Read the model definition and answer for the solid it produces. Units are mm, in the model's axes. Face numbers are marked on the shaded views. A direction names the side the tool comes from. Coordinates: 2 decimals unless noted, no trailing zeros. Loops run counter-clockwise (first coordinate to the right, second up) from the corner with the lowest first, then second, coordinate; pieces in that order, holes last. Notation, with made-up numbers: M 3,71 L 46,71 A26 cw 46,106 Z; hole C 1.25,68.5 d9. An arc over 180 degrees is marked long. One line per item, written item: value. Start each with the question number.
1. For the marked faces 1, 2 and 3, determine the directions among +Z, -Z, +X, -X, +Y, -Y from which every point of the face is accessible in a straight line to the end or side of a thin tool.
2. Flat-ended cylindrical pins translate along their axes: pin 1 (12 mm diameter, centred on x = -22.5, y = -18, fed in from +Z); pin 2 (19.5 mm diameter, centred on y = -15.5, z = -32.5, fed in from +X); pin 3 (5.5 mm diameter, centred on y = -21, z = -36.37, fed in from -X); pin 4 (20 mm diameter, centred on y = 21, z = -36.37, fed in from -X). Find the tip coordinate at first contact, or state that the pin passes through.
3. The part is cut by section C-C (x = -22.5). Write down the section's boundary in (y, z).
4. The part is cut by section A-A (x = 3). Write down the section's boundary in (y, z).
5. Consider probe 1 along Y at (x, z) = (9.5, 0); probe 2 along Z at (x, y) = (8, -14); probe 3 along X at (y, z) = (-10.5, -45.5). Determine where each line is inside the solid, lowest interval first.
6. The part is cut by section B-B (z = 0). State how many separate pieces and enclosed holes the cut face has, then the cut area to 3 significant figures.
7. Determine the mould class of the marked faces 4, 5 and 6 for opening direction Y: +Y half, -Y half, draft (parallel to the pull), parting line (faces both ways), or undercut.
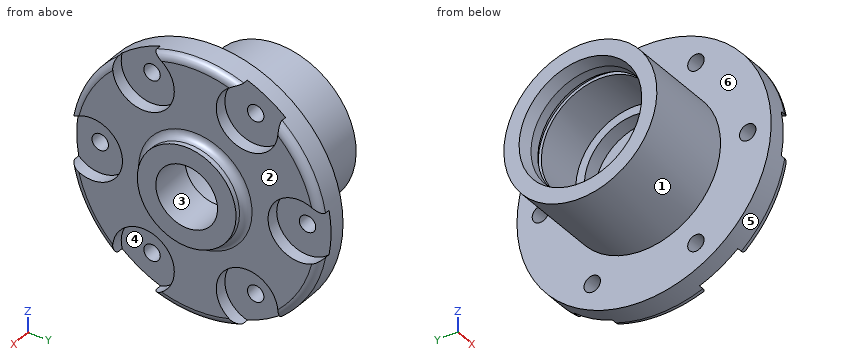
Autodesk Inventor part; units mm, degrees
ref_plane "Work Plane1" through (-26, 0, 0) normal (-1, 0, 0) x (0, 0, 1)
ref_plane "YZ Plane" through (0, 0, 0) normal (1, 0, 0) x (0, 1, 0)
ref_plane "XZ Plane" through (0, 0, 0) normal (0, 1, 0) x (-1, 0, 0)
sketch "Sketch1" plane through (0, 0, 0) normal (1, 0, 0) x (0, 1, 0)
  circle A0 centre (0, 0) radius 51.5
  circle A1 centre (0, 0) radius 31
  circle A2 centre (0, 0) radius 11
  dimension "d0" = 103
  dimension "d2" = 62
  dimension "d3" = 22
extrude "Extrusion1" add sketch "Sketch1" along normal blind 12 contours A0 | A1 | A2
sketch "Sketch3" plane through (0, 0, 0) normal (-1, 0, 0) x (0, 0, 1)
  circle A0 centre (0, 0) radius 11
  circle A1 centre (0, 0) radius 31
  dimension "d13" = 62
extrude "Extrusion2" add sketch "Sketch3" along normal blind 60 contours A0 | A1
sketch "Sketch4" plane through (12, 0, 0) normal (1, 0, 0) x (0, 0, -1)
  circle A0 centre (0, 0) radius 20
  dimension "d16" = 40
extrude "Extrusion3" add sketch "Sketch4" along normal blind 5
sketch "Sketch6" plane through (12, 0, 0) normal (1, 0, 0) x (0, 0, -1)
  circle A0 centre (0, 0) radius 11
  circle A1 centre (0, 0) radius 42
  line L0 (0, 0) -> (0, 42)
  point P0 (0.0095, 11)
  point P1 (0.0095, -11)
  point P2 (-36.3731, 21)
  point P3 (-36.3731, -21)
  point P4 (0, -42)
  point P5 (36.3731, -21)
  point P6 (36.3731, 21)
  dimension "d30" = 84
  dimension "d28" = 360
hole "Hole3" at (12, 42, 0) at (12, 21, 36.3731) at (12, -21, 36.3731) at (12, -42, 0) at (12, -21, -36.3731) at (12, 21, -36.3731) direction (-1, 0, 0) diameter 6.647 end through all counterbore diameter 25 counterbore depth 5
thread "Thread1"
sketch "Sketch7" plane through (17, 0, 0) normal (1, 0, 0) x (0, 0, -1)
  circle A0 centre (0, 0) radius 20
  circle A1 centre (0, 0) radius 12.5
  dimension "d40" = 25
extrude "Extrusion4" cut sketch "Sketch7" against normal blind 100 contours A1
fillet "Fillet1" radius 3 6 edges at (12, 44.6003, -25.75) (12, 0, -51.5) (12, -44.6003, -25.75) (12, -44.6003, 25.75) (12, 0, 51.5) (12, 44.6003, 25.75)
fillet "Fillet2" radius 3 1 edges at (12, 0, 20)
sketch "Sketch8" plane through (-60, 0, 0) normal (-1, 0, 0) x (0, 0, 1)
  circle A0 centre (0, 0) radius 23.5
  dimension "d45" = 47
extrude "Extrusion5" cut sketch "Sketch8" against normal blind 60
sketch "Sketch9" plane through (-60, 0, 0) normal (-1, 0, 0) x (0, 0, 1)
  circle A0 centre (0, 0) radius 11
  circle A1 centre (0, 0) radius 31
  circle A2 centre (0, 0) radius 31
extrude "Extrusion6" cut sketch "Sketch9" against normal blind 23 contours A0 | A1
chamfer "Chamfer1" distance 5 angle 15 1 edges at (-37, 0, -23.5) measured on face at (-12.3333, -1.891, 23.4238)
sketch "Sketch10" plane through (0, 0, 0) normal (-1, 0, 0) x (0, 0, 1)
  circle A0 centre (0, 0) radius 20
  circle A1 centre (0, 0) radius 23.5
  dimension "d60" = 40
extrude "Extrusion7" add sketch "Sketch10" along normal blind 6
ref_plane "Work Plane1" through (-26, 0, 0) normal (-1, 0, 0) x (0, 0, 1)
sketch "Sketch11" plane through (-26, 0, 0) normal (-1, 0, 0) x (0, 0, 1)
  circle A0 centre (0, 0) radius 24.75
  dimension "d64" = 49.5
extrude "Extrusion8" cut sketch "Sketch11" along normal blind 2
properties part number "END CAP" material "Iron, Cast"
Answer block:
1. face 1: -X
1. face 2: +X
1. face 3: +X, -X
2. pin 1: stops at z = 28.58
2. pin 2: stops at x = 12
2. pin 3: passes through
2. pin 4: stops at x = 0
3. outline: C 0,0 d62; hole C 0,0 d47
4. outline: C 0,0 d103; hole C -42,0 d6.65; hole C -21,-36.37 d6.65; hole C -21,36.37 d6.65; hole C 0,0 d25; hole C 21,-36.37 d6.65; hole C 21,36.37 d6.65; hole C 42,0 d6.65
5. probe 1: y = -29.5 to -12.5, 12.5 to 29.5
5. probe 2: z = -49.56 to -46.73, -26.02 to 26.02, 46.73 to 49.56
5. probe 3: x = 0 to 12
6. separate pieces: 4
6. enclosed holes: 0
6. area: 1,290 mm2
7. face 4: undercut
7. face 5: parting line
7. face 6: draft
